Geometry: see drawing. Coordinates: mm, zero at the bounding-box minimum. A direction names the side the tool comes from. Give positions to 0.01 mm unless a question says otherwise; leave off trailing zeros. Write each loop counter-clockwise with the first axis right and the second up, starting at its lowest first coordinate (ties: lowest second). Pieces come first, ordered by that corner, then holes. Notation, with made-up numbers: (-10, -32) -> (49, -32) arc R18 ccw to (49, -25) -> close; hole circle Ø2 at (-35, 29.25). An arc over 180 degrees is marked (long way). Answer as a JSON object with one key per item and string values. Group by question number.
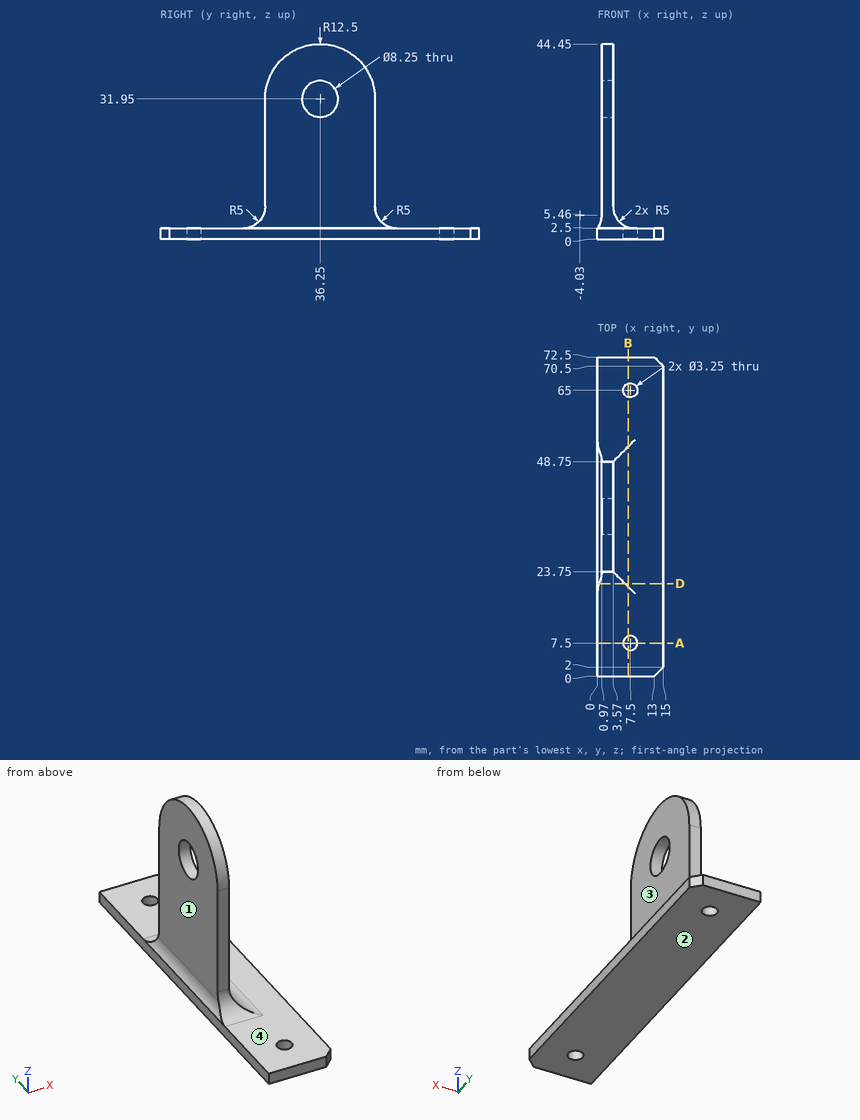
1. Contact query for flat-ended pins moving along their axis: pin 1 Ø8 at (x, y) = (3.5, 17) entering from +Z (1 decimal); pin 2 Ø8 at (x, y) = (7, 24) entering from -Z; pin 3 Ø4.5 at (x, y) = (8, 41.5) entering from +Z; pin 4 Ø9.5 at (y, z) = (36.25, 31.95) entering from -X. Output: stop coordinate, or through.
2. Section B-B (x = 7). Return the cut outline in (y, z).
3. Section D-D (y = 21). Return the cut outline in (x, z) (1 decimal).
4. Section A-A (y = 7.5). Return the cut outline in (x, z) (1 decimal).
5. Line query: line 1 (Y direction, x = 7.5, z = 0.8) (1 decimal); line 2 (X direction, y = 65, z = 1.55) (1 decimal); line 3 (Z direction, x = 10, y = 5). Output: solid intervals per line, ascending.
6. Reachability of the marked faces 1, 2, 3 and 4 from +Z, -Z, +X, -X, +Y, -Y: full face, straight path, thin tool, end or side. Return the list, or none.
Working result:
{
 "1": {"pin 1": "stops at z = 3", "pin 2": "stops at z = 0", "pin 3": "stops at z = 3.37", "pin 4": "stops at x = 0.97"},
 "2": {"outline": "(0, 0) -> (5.95, 0) -> (5.95, 2.5) -> (0, 2.5) -> close; (9.05, 0) -> (63.45, 0) -> (63.45, 2.5) -> (53.75, 2.5) arc R5 cw to (52.18, 2.75) -> (20.32, 2.75) arc R5 cw to (18.75, 2.5) -> (9.05, 2.5) -> close; (66.55, 0) -> (72.5, 0) -> (72.5, 2.5) -> (66.55, 2.5) -> close"},
 "3": {"outline": "(0, 0) -> (15, 0) -> (15, 2.5) -> (8.6, 2.5) arc R5 cw to (6.3, 3) -> (0.3, 3) arc R5 cw to (0, 2.5) -> close"},
 "4": {"outline": "(0, 0) -> (5.9, 0) -> (5.9, 2.5) -> (0, 2.5) -> close; (9.1, 0) -> (15, 0) -> (15, 2.5) -> (9.1, 2.5) -> close"},
 "5": {"line 1": "y = 0 to 5.9, 9.1 to 63.4, 66.6 to 72.5", "line 2": "x = 0 to 5.9, 9.1 to 15", "line 3": "z = 0 to 2.5"},
 "6": {"face 1": "+Z, -X, +Y, -Y", "face 2": "-Z, +X, -X, +Y, -Y", "face 3": "+Z, +X, +Y, -Y", "face 4": "+Z, +X"}
}
